Model file for the job. Use its own axes, mm. A direction names the side the tool comes from. Coordinates: 2 decimals unless noted, no trailing zeros. Order: outer loops, then holes, each group sorted by start corner. A loop starts at its lowest first (then second) coordinate and runs counter-clockwise, first axis right, second up. Notation, with made-up numbers: (9, -23.75) -> (14, -23.75) arc R28 cw to (14, 5.25) -> close; hole circle Ø6 at (72.25, -35.5). An arc over 180 degrees is marked (long way). Use CSV: the item, a comma, the result in double quotes. Start each with the question number.
(1) Tool access for faces 1 (the flat face through (0, 2, 13)), 2 (the flat face through (-17.1, 27, 29)), 3 (the flat face through (-22, 51, 29)): list every direction of +Z, -Z, +X, -X, +Y, -Y with a clear straight run to the whole face (end or side of a thin tool).
(2) Cut at C-C on x = 0. Write the cut outline in (y, z), plus the area to 3 significant figures.
(3) Pin check, flat tips, straight feed: pin 1 Ø4 at (x, z) = (-15.5, 15.5) entering from +Y; pin 2 Ø3 at (x, z) = (-4.5, -9.5) entering from -Y; pin 3 Ø6 at (x, y) = (12, 5.5) entering from -Z; pin 4 Ø14.5 at (x, y) = (-9, 26.5) entering from -Z. Stop position of each tip, or through.
(4) Cut at D-D on y = 24. Write the cut outline in (x, z).
(5) Probe L1, parallel to X at y = 0.5, z = 15.5; L2, parallel to X at y = 0.8, z = 0; L3, parallel to Z at x = -2.5, y = 23. List the from-to ranges inside material, lowest first.
(6) Cut at A-A on z = 0. Write the cut outline in (x, y).
(7) Cut at B-B on y = 15. Write the cut outline in (x, z).
(8) Pull direction Y, two halves, no side cores. Call faces 4 (the flat face through (-23.99, 12.14, 21.59)), 5 (the cylindrical face through (-15, 44.1, 29)), 6 (the cylindrical face through (-15, 9.9, 29)), 7 (the cylindrical face through (17, 1, -14.6)): pulls with the +Y half, pulls with the -Y half, needs draft (parallel to the pull), parting line crosses it, or undercut.
```python
from build123d import *

# Parameters (mm, degrees)
SKETCH_1_W               = 50
SKETCH_1_H               = 49
SKETCH_1_R               = 11.05
SKETCH_1_R_2             = 1.75
EXTRUDE_1_DEPTH          = 2
CHAMFER_1_SIZE           = 5
SKETCH_3_W               = 50
SKETCH_3_H               = 2
EXTRUDE_2_DEPTH          = 53
CHAMFER_2_SIZE           = 5
CHAMFER_3_SIZE           = 5
CUT_EXTRUDE_1_DEPTH      = 77.387171698
CUT_EXTRUDE_1_DEPTH_BACK = 77.387171698
RIB_1_REACH              = 80.797
SKETCH_5_WALL_W          = 183.448137028
SKETCH_5_WALL_H          = 2
FILLET_1_R               = 2


with BuildPart() as part:
    # 草图1 → 凸台-拉伸1 (new body)
    with BuildSketch(Plane(origin=(0, 0, 0), x_dir=(1, 0, 0), z_dir=(0, 1, 0))):
        with Locations((0, -3.5)):
            Rectangle(SKETCH_1_W, SKETCH_1_H)
        with Locations(Location((0, 0, 0), (0, 0, 270))):
            Circle(SKETCH_1_R, mode=Mode.SUBTRACT)
        with Locations(Location((15.5, 15.5, 0), (0, 0, 270))):
            Circle(SKETCH_1_R_2, mode=Mode.SUBTRACT)
        with Locations(Location((15.5, -15.5, 0), (0, 0, 90))):
            Circle(SKETCH_1_R_2, mode=Mode.SUBTRACT)
        with Locations(Location((-15.5, -15.5, 0), (0, 0, 270))):
            Circle(SKETCH_1_R_2, mode=Mode.SUBTRACT)
        with Locations(Location((-15.5, 15.5, 0), (0, 0, 90))):
            Circle(SKETCH_1_R_2, mode=Mode.SUBTRACT)
    extrude(amount=EXTRUDE_1_DEPTH)

    # 倒角1
    chamfer_1_edges = [part.edges().sort_by_distance(p)[0] for p in [
        (-25, 1, -21),
        (25, 1, -21),
    ]]
    chamfer(chamfer_1_edges, length=CHAMFER_1_SIZE)

    # 草图3 → 凸台-拉伸2 (add)
    with BuildSketch(Plane(origin=(0, 0, 0), x_dir=(1, 0, 0), z_dir=(0, 1, 0))):
        with Locations((0, -29)):
            Rectangle(SKETCH_3_W, SKETCH_3_H)
    extrude(amount=EXTRUDE_2_DEPTH)

    # 倒角2
    chamfer_2_edges = [part.edges().sort_by_distance(p)[0] for p in [
        (-25, 53, 29),
    ]]
    chamfer(chamfer_2_edges, length=CHAMFER_2_SIZE)

    # 倒角3
    chamfer_3_edges = [part.edges().sort_by_distance(p)[0] for p in [
        (25, 53, 29),
    ]]
    chamfer(chamfer_3_edges, length=CHAMFER_3_SIZE)

    # 草图4 → 切除-拉伸1 (cut, two sides: drawn at the far end of the back side and taken through both)
    with BuildSketch(Plane(origin=(0, 0, 28), x_dir=(-1, 0, 0), z_dir=(0, 0, -1)).offset(-CUT_EXTRUDE_1_DEPTH_BACK)):
        with BuildLine():
            Line((-17.1, 42), (-17.1, 12))
            ThreePointArc((-17.1, 12), (-15, 9.9), (-12.9, 12))
            Line((-12.9, 12), (-12.9, 42))
            ThreePointArc((-12.9, 42), (-15, 44.1), (-17.1, 42))
        make_face()
        with BuildLine():
            ThreePointArc((17.1, 12), (15, 9.9), (12.9, 12))
            Line((12.9, 12), (12.9, 42))
            ThreePointArc((12.9, 42), (15, 44.1), (17.1, 42))
            Line((17.1, 42), (17.1, 12))
        make_face()
    extrude(amount=CUT_EXTRUDE_1_DEPTH + CUT_EXTRUDE_1_DEPTH_BACK, mode=Mode.SUBTRACT)

    # 草图5 wall → 筋1 (add, up to next)
    with BuildSketch(Plane(origin=(25, 12, 21.5), x_dir=(0, -0.838443616301, -0.544988350595), z_dir=(0, 0.544988350595, -0.838443616301)), mode=Mode.PRIVATE) as rib_1_sk1:
        with Locations((0, 1)):
            Rectangle(SKETCH_5_WALL_W, SKETCH_5_WALL_H)
    rib_1_tool1 = extrude(rib_1_sk1.sketch, amount=-RIB_1_REACH, mode=Mode.PRIVATE) - part.part
    rib_1 = rib_1_tool1.solids().sort_by_distance((25, 12, 21.5))[0]
    add(rib_1)

    # 镜向1: 筋1 across plane
    add(rib_1.mirror(Plane(origin=(0, 0, 0), x_dir=(0, 0, 1), z_dir=(1, 0, 0))))

    # 圆角1
    fillet_1_edges = [part.edges().sort_by_distance(p)[0] for p in [
        (0, 2, 28),
    ]]
    fillet(fillet_1_edges, radius=FILLET_1_R)


solid = part.part
```
Outcome:
1,face 1,"-Z, +Y"
1,face 2,"+Z, -Z"
1,face 3,"+Z, -Z, -X, +Y"
2,outline,"(0, -21) -> (2, -21) -> (2, -11.05) -> (0, -11.05) -> close; (0, 11.05) -> (2, 11.05) -> (2, 26) arc R2 cw to (4, 28) -> (53, 28) -> (53, 30) -> (0, 30) -> close"
2,area,"161 mm2"
3,pin 1,"y = 2"
3,pin 2,"y = 0"
3,pin 3,"z = 27.32"
3,pin 4,"z = 28"
4,outline,"(-25, 28) -> (-17.1, 28) -> (-17.1, 30) -> (-25, 30) -> close; (-12.9, 28) -> (12.9, 28) -> (12.9, 30) -> (-12.9, 30) -> close; (17.1, 28) -> (25, 28) -> (25, 30) -> (17.1, 30) -> close"
5,L1,"-25 to -17.25, -13.75 to 13.75, 17.25 to 25"
5,L2,"-25 to -11.05, 11.05 to 25"
5,L3,"28 to 30"
6,outline,"(-25, 0) -> (-11.05, 0) -> (-11.05, 2) -> (-25, 2) -> close; (11.05, 0) -> (25, 0) -> (25, 2) -> (11.05, 2) -> close"
7,outline,"(-25, 23.45) -> (-23, 23.45) -> (-23, 28) -> (-17.1, 28) -> (-17.1, 30) -> (-25, 30) -> close; (-12.9, 28) -> (12.9, 28) -> (12.9, 30) -> (-12.9, 30) -> close; (17.1, 28) -> (23, 28) -> (23, 23.45) -> (25, 23.45) -> (25, 30) -> (17.1, 30) -> close"
8,face 4,"pulls with the +Y half"
8,face 5,"undercut"
8,face 6,"undercut"
8,face 7,"needs draft"
